from build123d import *

# Parameters (mm, degrees)
SKETCH1_W               = 190.5
SKETCH1_H               = 152.4
BOSS_EXTRUDE1_DEPTH     = 6.35
SKETCH2_W               = 12.7
SKETCH2_H               = 6.35
CUT_EXTRUDE1_DEPTH      = 7.35
LPATTERN1_COUNT         = 7
LPATTERN1_PITCH         = 25.4
SKETCH3_W               = 6.35
SKETCH3_H               = 12.7
CUT_EXTRUDE2_DEPTH      = 7.35
LPATTERN2_COUNT         = 6
LPATTERN2_PITCH         = 25.4
MIRROR2_COPY_1_SKETCH_W = 6.35
MIRROR2_COPY_1_SKETCH_H = 12.7
MIRROR2_COPY_1_DEPTH    = 7.35
MIRROR2_COPY_2_SKETCH_W = 6.35
MIRROR2_COPY_2_SKETCH_H = 12.7
MIRROR2_COPY_2_DEPTH    = 7.35
MIRROR2_COPY_3_SKETCH_W = 6.35
MIRROR2_COPY_3_SKETCH_H = 12.7
MIRROR2_COPY_3_DEPTH    = 7.35
MIRROR2_COPY_4_SKETCH_W = 6.35
MIRROR2_COPY_4_SKETCH_H = 12.7
MIRROR2_COPY_4_DEPTH    = 7.35
MIRROR2_COPY_5_SKETCH_W = 6.35
MIRROR2_COPY_5_SKETCH_H = 12.7
MIRROR2_COPY_5_DEPTH    = 7.35
SKETCH4_W               = 12.7
SKETCH4_H               = 6.35
CUT_EXTRUDE3_DEPTH      = 7.35
LPATTERN3_COUNT         = 7
LPATTERN3_PITCH         = 25.4


with BuildPart() as part:
    # Sketch1 → Boss-Extrude1 (new body)
    with BuildSketch(Plane.XY):
        Rectangle(SKETCH1_W, SKETCH1_H)
    extrude(amount=BOSS_EXTRUDE1_DEPTH)

    # Sketch2 → Cut-Extrude1 (cut, through all)
    with BuildSketch(Plane.XY.offset(6.35)):
        with Locations((-69.85, 73.025)):
            Rectangle(SKETCH2_W, SKETCH2_H)
    cut_extrude1 = extrude(amount=-CUT_EXTRUDE1_DEPTH, mode=Mode.SUBTRACT)

    # LPattern1: Cut-Extrude1 ×7
    with Locations(*[(i * LPATTERN1_PITCH, 0, 0) for i in range(1, LPATTERN1_COUNT)]):
        add(cut_extrude1, mode=Mode.SUBTRACT)

    # Sketch3 → Cut-Extrude2 (cut, through all)
    with BuildSketch(Plane.XY.offset(6.35)):
        with Locations((92.075, 69.85)):
            Rectangle(SKETCH3_W, SKETCH3_H)
    cut_extrude2 = extrude(amount=-CUT_EXTRUDE2_DEPTH, mode=Mode.SUBTRACT)

    # LPattern2: Cut-Extrude2 ×6
    with Locations(*[(0, -i * LPATTERN2_PITCH, 0) for i in range(1, LPATTERN2_COUNT)]):
        add(cut_extrude2, mode=Mode.SUBTRACT)

    # Mirror2: Cut-Extrude2 across plane
    add(cut_extrude2.mirror(Plane(origin=(0, 0, 0), x_dir=(0, 0, 1), z_dir=(1, 0, 0))), mode=Mode.SUBTRACT)

    # Mirror2 copy 1 sketch → Mirror2 copy 1 (cut, through all)
    with BuildSketch(Plane(origin=(0, -25.4, 6.35), x_dir=(-1, 0, 0), z_dir=(0, 0, 1))):
        with Locations((92.075, -69.85)):
            Rectangle(MIRROR2_COPY_1_SKETCH_W, MIRROR2_COPY_1_SKETCH_H)
    extrude(amount=-MIRROR2_COPY_1_DEPTH, mode=Mode.SUBTRACT)

    # Mirror2 copy 2 sketch → Mirror2 copy 2 (cut, through all)
    with BuildSketch(Plane(origin=(0, -50.8, 6.35), x_dir=(-1, 0, 0), z_dir=(0, 0, 1))):
        with Locations((92.075, -69.85)):
            Rectangle(MIRROR2_COPY_2_SKETCH_W, MIRROR2_COPY_2_SKETCH_H)
    extrude(amount=-MIRROR2_COPY_2_DEPTH, mode=Mode.SUBTRACT)

    # Mirror2 copy 3 sketch → Mirror2 copy 3 (cut, through all)
    with BuildSketch(Plane(origin=(0, -76.2, 6.35), x_dir=(-1, 0, 0), z_dir=(0, 0, 1))):
        with Locations((92.075, -69.85)):
            Rectangle(MIRROR2_COPY_3_SKETCH_W, MIRROR2_COPY_3_SKETCH_H)
    extrude(amount=-MIRROR2_COPY_3_DEPTH, mode=Mode.SUBTRACT)

    # Mirror2 copy 4 sketch → Mirror2 copy 4 (cut, through all)
    with BuildSketch(Plane(origin=(0, -101.6, 6.35), x_dir=(-1, 0, 0), z_dir=(0, 0, 1))):
        with Locations((92.075, -69.85)):
            Rectangle(MIRROR2_COPY_4_SKETCH_W, MIRROR2_COPY_4_SKETCH_H)
    extrude(amount=-MIRROR2_COPY_4_DEPTH, mode=Mode.SUBTRACT)

    # Mirror2 copy 5 sketch → Mirror2 copy 5 (cut, through all)
    with BuildSketch(Plane(origin=(0, -127, 6.35), x_dir=(-1, 0, 0), z_dir=(0, 0, 1))):
        with Locations((92.075, -69.85)):
            Rectangle(MIRROR2_COPY_5_SKETCH_W, MIRROR2_COPY_5_SKETCH_H)
    extrude(amount=-MIRROR2_COPY_5_DEPTH, mode=Mode.SUBTRACT)

    # Sketch4 → Cut-Extrude3 (cut, through all)
    with BuildSketch(Plane.XY.offset(6.35)):
        with Locations((-76.2, -73.025)):
            Rectangle(SKETCH4_W, SKETCH4_H)
    cut_extrude3 = extrude(amount=-CUT_EXTRUDE3_DEPTH, mode=Mode.SUBTRACT)

    # LPattern3: Cut-Extrude3 ×7
    with Locations(*[(i * LPATTERN3_PITCH, 0, 0) for i in range(1, LPATTERN3_COUNT)]):
        add(cut_extrude3, mode=Mode.SUBTRACT)


solid = part.part
Model file for the job. Use its own axes, mm. A direction names the side the tool comes from. Give positions to 0.01 mm unless a question says otherwise; leave off trailing zeros. Loops run counter-clockwise (first coordinate to the right, second up) from the corner with the lowest first, then second, coordinate; pieces in that order, holes last. Notation, with made-up numbers: (-8, -11.5) - (29, -11.5) arc R37 ccw to (29, 25.5) - close; hole circle Ø7 at (0.25, 69). An arc over 180 degrees is marked (long way). Use one line per item in the form item = value.
(1) Cut at A-A (y = -4.5). Give the cut face in (x, z), then the cut area to 3 significant figures.
Determined:
outline = (-88.9, 0) - (88.9, 0) - (88.9, 6.35) - (-88.9, 6.35) - close
area = 1,130 mm^2
(2) Drill centre lines: L1, parallel to X at y = -51, z = 4; L2, parallel to Y at x = 20, z = 1.5; L3, parallel to Y at x = -67, z = 4.75. Where is each one in solid material? Low to high.
Determined:
L1 = -88.9 to 88.9
L2 = -69.85 to 76.2
L3 = -76.2 to 69.85
(3) Pull direction Y, two halves, no side cores. Call faces 6 (the face through (-6, 76.2, 3)), 7 (the face through (-1, 1, 0)), 8 (the face through (88.9, -6, 3)): pulls with the +Y half, pulls with the -Y half, needs draft (parallel to the pull), parting line crosses it, or undercut.
Determined:
face_6 = pulls with the +Y half
face_7 = needs draft
face_8 = undercut
(4) 3-axis set-ups, long thin cutter, end or side, ignore diameter. For faces 1 (the face through (19.05, -73, 3)), 2 (the face through (-25.4, 73, 3)), 3 (the face through (92, -12.7, 3)), 4 (the face through (19, 76.2, 3)), 5 (the face through (-92, 25.4, 3)): which of +Z, -Z, +X, -X, +Y, -Y reach the whole face in a straight line?
Determined:
face_1 = +Z, -Z, -Y
face_2 = +Z, -Z, +Y
face_3 = +Z, -Z, +X
face_4 = +Z, -Z, +X, -X, +Y
face_5 = +Z, -Z, -X
(5) Cut at B-B (x = 54). Give the cut face in (y, z).
Determined:
outline = (-69.85, 0) - (69.85, 0) - (69.85, 6.35) - (-69.85, 6.35) - close
(6) Drop flat-ended pins along their axis: P1, Ø10, axis at x = -36.5, y = -31, coming from the -Z side; P2, Ø3, axis at x = -76.5, z = 2, coming from the -Y side; P3, Ø1.9, axis at y = 21, z = 2.5, coming from the -X side; P4, Ø2, axis at x = 54.5, z = 3, coming from the +Y side. Give the stop position or say it passes through.
Determined:
P1 = 0
P2 = -69.85
P3 = -88.9
P4 = 69.85
